Part model, mm, in its own coordinate system. A direction names the side the tool comes from. Coordinates: 2 decimals unless noted, no trailing zeros. Write each loop counter-clockwise with the first axis right and the second up, starting at its lowest first coordinate (ties: lowest second). Pieces come first, ordered by that corner, then holes. Notation, with made-up numbers: (64.5, 81.5) - (105.5, 81.5) arc R20 cw to (105.5, 110.5) - close; hole circle Ø7 at (38.25, 79). An arc over 180 degrees is marked (long way). Use a Markdown table: item, result.
Autodesk Inventor part; units mm, degrees
ref_plane "YZ Plane" through (0, 0, 0) normal (1, 0, 0) x (0, 1, 0)
ref_plane "XZ Plane" through (0, 0, 0) normal (0, 1, 0) x (-1, 0, 0)
ref_plane "XY Plane" through (0, 0, 0) normal (0, 0, 1) x (1, 0, 0)
sketch "Эскиз1" plane through (0, 0, 0) normal (0, 0, 1) x (1, 0, 0)
  line L0 (8.5, -8.5) -> (-8.5, -8.5)
  line L1 (8.5, 8.5) -> (8.5, -8.5)
  line L2 (-8.5, -8.5) -> (-8.5, 8.5)
  line L3 (-8.5, 8.5) -> (8.5, 8.5)
  line L4 (-6.5, -6.5) -> (6.5, -6.5)
  line L5 (6.5, -6.5) -> (6.5, 6.5)
  line L6 (6.5, 6.5) -> (-6.5, 6.5)
  line L7 (-6.5, 6.5) -> (-6.5, -6.5)
  point P0 (0, 0)
  dimension "d0" = 2
extrude "Выдавливание1" add sketch "Эскиз1" against normal blind 10
sketch "Эскиз2" plane through (0, 0, 0) normal (0, 0, 1) x (1, 0, 0)
  line L0 (13, -13.5) -> (-13.5, -13.5)
  line L1 (13, 13) -> (13, -13.5)
  line L2 (-13.5, 13) -> (13, 13)
  line L3 (-13.5, -13.5) -> (-13.5, 13)
  point P0 (0, 0)
extrude "Выдавливание2" add sketch "Эскиз2" along normal blind 5
fillet "Сопряжение1" radius 2 4 edges at (8.5, 8.5, -5) (-8.5, 8.5, -5) (-8.5, -8.5, -5) (8.5, -8.5, -5)
fillet "Сопряжение2" radius 4 4 edges at (-13.5, -13.5, 2.5) (13, -13.5, 2.5) (13, 13, 2.5) (-13.5, 13, 2.5)
ref_plane "РабПлоскость2" through (-9.5, 4.75, 0) normal (0, 1, 0) x (1, 0, 0)
ref_plane "РабПлоскость1" through (-9.5, -0.25, 0) normal (0, 1, 0) x (1, 0, 0)
sketch "Эскиз3" plane through (-9.5, 4.75, 0) normal (0, 1, 0) x (1, 0, 0)
  line L0 (0, -5) -> (18.5, -5)
  line L1 (2.3593, -5) -> (4.8015, -11.7101)
  line L2 (16.6407, -5) -> (14.1985, -11.7101)
  arc A0 (4.8015, -11.7101) -> (14.1985, -11.7101) centre (9.5, -10) ccw
  circle A1 centre (9.5, -10) radius 2
  line L3 (16, 10) -> (3, 10)
  line L4 (0, -5) -> (-4, -5)
  point P0 (9.5, 0)
  point P1 (9.5, 10)
  dimension "d10" = 4
  dimension "d11" = 5
  dimension "d12" = 5
  dimension "d13" = 70
extrude "Выдавливание3" add sketch "Эскиз3" along normal blind 4
properties part number "cum_holder_down"
Item 1: Which spindle directions (+Z, -Z, +X, -X, +Y, -Y) get a long thin tool onto all of the face, cutting with end or side? Do faces 4 (the face through (0, 6.5, -5)), 5 (the face through (-0.1, 4.75, 7.7)), 6 (the face through (7.9, 7.93, -5.07)), 7 (the face through (7.93, -7.9, -5.07)), 8 (the face through (-0.1, 8.75, 7.7)). Say none if no direction does.
From the geometry:
| item | result |
|---|---|
| face 4 | -Z |
| face 5 | +Z, +X, -X, -Y |
| face 6 | -Z, +X, +Y |
| face 7 | -Z, +X, -Y |
| face 8 | +Z, +X, -X, +Y |
Item 2: Drill centre lines: probe 1 along X at (y, z) = (-3.25, -5.75); probe 2 along Z at (x, y) = (0, 7.35); probe 3 along Z at (x, y) = (0, 5.6). Where is each one in solid material? Low to high.
From the geometry:
| item | result |
|---|---|
| probe 1 | -8.5 to -6.5, 6.5 to 8.5 |
| probe 2 | -10 to 8, 12 to 15 |
| probe 3 | 0 to 8, 12 to 15 |
Item 3: Band-saw the part on C-C, the plane y = 5.5. Give the cut face in (x, z), then the cut area to 3 significant figures.
From the geometry:
| item | result |
|---|---|
| outline | (-13.5, 0) - (-8.5, 0) - (-8.5, -10) - (-6.5, -10) - (-6.5, 0) - (6.5, 0) - (6.5, -10) - (8.5, -10) - (8.5, 0) - (13, 0) - (13, 5) - (7.14, 5) - (4.7, 11.71) arc R5 ccw to (-4.7, 11.71) - (-7.14, 5) - (-13.5, 5) - close; hole circle Ø4 at (0, 10) |
| area | 262 mm^2 |
Item 4: Band-saw the part on B-B, the plane z = -7. Give the cut face in (x, y).
From the geometry:
| item | result |
|---|---|
| outline | (-8.5, -6.5) arc R2 ccw to (-6.5, -8.5) - (6.5, -8.5) arc R2 ccw to (8.5, -6.5) - (8.5, 6.5) arc R2 ccw to (6.5, 8.5) - (-6.5, 8.5) arc R2 ccw to (-8.5, 6.5) - close; hole (-6.5, -6.5) - (6.5, -6.5) - (6.5, 6.5) - (-6.5, 6.5) - close |
Item 5: Band-saw the part on D-D, the plane z = 11. Give the cut face in (x, y).
From the geometry:
| item | result |
|---|---|
| outline | (-4.96, 4.75) - (-1.73, 4.75) - (-1.73, 8.75) - (-4.96, 8.75) - close; (1.73, 4.75) - (4.96, 4.75) - (4.96, 8.75) - (1.73, 8.75) - close |
Item 6: Two-plate mould, pull along X, no slides. Class faces 1 (the face through (0, 7, 12)), 2 (the face through (-8, 0, -10)), 3 (the face through (0, 7, 15)): pulls with the +X half, pulls with the -X half, needs draft (parallel to the pull), parting line crosses it, or undercut.
From the geometry:
| item | result |
|---|---|
| face 1 | undercut |
| face 2 | needs draft |
| face 3 | parting line crosses it |
Item 7: Band-saw the part on A-A, the plane x = 0. Give the cut face in (y, z).
From the geometry:
| item | result |
|---|---|
| outline | (-13.5, 0) - (-8.5, 0) - (-8.5, -10) - (-6.5, -10) - (-6.5, 0) - (6.5, 0) - (6.5, -10) - (8.5, -10) - (8.5, 0) - (13, 0) - (13, 5) - (8.75, 5) - (8.75, 8) - (4.75, 8) - (4.75, 5) - (-13.5, 5) - close; (4.75, 12) - (8.75, 12) - (8.75, 15) - (4.75, 15) - close |
Item 8: Drop flat-ended pins along their axis: P1, Ø3, axis at y = 0, z = -6.5, coming from the -X side; P2, Ø6, axis at x = -6.5, y = -0.5, coming from the +Z side; P3, Ø4, axis at x = 6.5, z = 9, coming from the -Y side. Give the stop position or say it passes through.
From the geometry:
| item | result |
|---|---|
| P1 | x = -8.5 |
| P2 | z = 5 |
| P3 | y = 4.75 |
